Build history of the part. All positions in model axes, mm. Round coordinates to 2 decimals unless told otherwise and drop trailing zeros. Order: outer loops, then holes, each group sorted by start corner. A loop starts at its lowest first (then second) coordinate and runs counter-clockwise, first axis right, second up. Notation, with made-up numbers: (28, 81) -> (77, 81) arc R31 cw to (77, 114) -> close; hole circle Ø5 at (82.5, -13). An arc over 180 degrees is marked (long way). Write item = value, one per line.
from build123d import *

# Parameters (mm, degrees)
BOSS_EXTRUDE1_DEPTH = 10
SKETCH3_R           = 4
CUT_EXTRUDE1_DEPTH  = 10


with BuildPart() as part:
    # Sketch2 → Boss-Extrude1 (new body)
    with BuildSketch(Plane.XY):
        with BuildLine():
            Line((25, 0), (25, 150))
            ThreePointArc((25, 150), (0, 175), (-25, 150))
            Line((-25, 150), (-25, 0))
            ThreePointArc((-25, 0), (0, -25), (25, 0))
        make_face()
    extrude(amount=BOSS_EXTRUDE1_DEPTH)

    # Sketch3 → Cut-Extrude1 (cut)
    with BuildSketch(Plane(origin=(0, 0, 0), x_dir=(-1, 0, 0), z_dir=(0, 0, -1))):
        Circle(SKETCH3_R)
    extrude(amount=-CUT_EXTRUDE1_DEPTH, mode=Mode.SUBTRACT)


solid = part.part
Q1. Cut at C-C, the plane x = -20. List the corners of the cut face in (y, z), and give its area (3 significant figures).
Check values:
outline = (-15, 0) -> (165, 0) -> (165, 10) -> (-15, 10) -> close
area = 1,800 mm²
Q2. Cut at B-B, the plane z = 3.75. List the corners of the cut face in (x, y), and give its area (3 significant figures).
Check values:
outline = (-25, 0) arc R25 ccw to (25, 0) -> (25, 150) arc R25 ccw to (-25, 150) -> close; hole circle Ø8 at (0, 0)
area = 9,410 mm²
Q3. Cut at A-A, the plane x = 0. List the corners of the cut face in (y, z), and give its area (3 significant figures).
Check values:
outline = (-25, 0) -> (-4, 0) -> (-4, 10) -> (-25, 10) -> close; (4, 0) -> (175, 0) -> (175, 10) -> (4, 10) -> close
area = 1,920 mm²
Q4. Cut at D-D, the plane y = 162.5. List the corners of the cut face in (x, z), and give its area (3 significant figures).
Check values:
outline = (-21.65, 0) -> (21.65, 0) -> (21.65, 10) -> (-21.65, 10) -> close
area = 433 mm²
Q5. Flat gauge pins, fed straight in: pin 1 (4 mm diameter, centred on x = -10, y = 31, fed in from -Z); pin 2 (6 mm diameter, centred on x = -10.5, z = 3, fed in from -Y); pin 3 (6.5 mm diameter, centred on x = 0, y = 0, fed in from -Z); pin 4 (3 mm diameter, centred on x = 12, z = 2.5, fed in from +Y). Where does each tip first touch, or does it go through?
Check values:
pin_1 = 0
pin_2 = -23.85
pin_3 = through
pin_4 = 172.69
Q6. Mould opens along Y. For faces 1 (the face through (0, 76, 10)), 2 (the face through (0.55, 174.994, 4.93)), 3 (the face through (0.867, -3.905, 4.93)) say: released by +Y, released by -Y, zero draft, split by the parting line, or undercut.
Check values:
face_1 = zero draft
face_2 = released by +Y
face_3 = undercut
Q7. Probe probe 1 along Y at (x, z) = (0, 3.75); probe 2 along Y at (x, z) = (-1, 8.5); probe 3 along Y at (x, z) = (-9, 7.75). List the from-to ranges inside material, lowest first.
Check values:
probe_1 = -25 to -4, 4 to 175
probe_2 = -24.98 to -3.87, 3.87 to 174.98
probe_3 = -23.32 to 173.32
